from build123d import *

# Parameters (mm, degrees)
SKETCH3_W                                    = 145.5000011
SKETCH3_H                                    = 83.82
BOSS_EXTRUDE1_DEPTH                          = 83.82
SKETCH4_W                                    = 141.50000148
SKETCH4_H                                    = 79.312008
CUT_EXTRUDE1_DEPTH                           = 71.882
CBORE_FOR_M3_HEX_HEAD_CAP_SCREW1_D           = 3.4
CBORE_FOR_M3_HEX_HEAD_CAP_SCREW1_DEPTH       = 3.99999962
CBORE_FOR_M3_HEX_HEAD_CAP_SCREW1_CBORE_D     = 9.351
CBORE_FOR_M3_HEX_HEAD_CAP_SCREW1_CBORE_DEPTH = 2
CUT_EXTRUDE3_REACH                           = 147.5
SKETCH5_R                                    = 12.7
CBORE_FOR_M3_HEX_HEAD_CAP_SCREW2_D           = 3.4
CBORE_FOR_M3_HEX_HEAD_CAP_SCREW2_DEPTH       = 4.507992
CBORE_FOR_M3_HEX_HEAD_CAP_SCREW2_CBORE_D     = 9.351
CBORE_FOR_M3_HEX_HEAD_CAP_SCREW2_CBORE_DEPTH = 2
F_3_0MM_DOWEL_HOLE1_D                        = 3
F_3_0MM_DOWEL_HOLE1_DEPTH                    = 4.507992
F_3_0MM_DOWEL_HOLE2_D                        = 3
F_3_0MM_DOWEL_HOLE2_DEPTH                    = 11.938
CBORE_FOR_M3_HEX_HEAD_CAP_SCREW3_D           = 3.4
CBORE_FOR_M3_HEX_HEAD_CAP_SCREW3_DEPTH       = 11.938
CBORE_FOR_M3_HEX_HEAD_CAP_SCREW3_CBORE_D     = 9.351
CBORE_FOR_M3_HEX_HEAD_CAP_SCREW3_CBORE_DEPTH = 2
SKETCH22_R                                   = 41.75000032
BOSS_EXTRUDE3_DEPTH                          = 170
SKETCH26_R                                   = 36.75001032
CUT_EXTRUDE5_DEPTH                           = 170
SKETCH27_W                                   = 141.50000148
SKETCH27_H                                   = 4.507992
CUT_EXTRUDE7_DEPTH                           = 71.882
SKETCH28_W                                   = 132.727764313
SKETCH28_H                                   = 83.82
CUT_EXTRUDE8_DEPTH                           = 6.35
TAP_DRILL_FOR_M6_TAP2_D                      = 5


with BuildPart() as part:
    # Sketch3 → Boss-Extrude1 (new body)
    with BuildSketch(Plane(origin=(0, 0, 0), x_dir=(1, 0, 0), z_dir=(0, 1, 0))):
        with Locations((33.920258223, -7.464260839)):
            Rectangle(SKETCH3_W, SKETCH3_H)
    extrude(amount=BOSS_EXTRUDE1_DEPTH)

    # Sketch4 → Cut-Extrude1 (cut)
    with BuildSketch(Plane(origin=(0, 83.82, 0), x_dir=(1, 0, 0), z_dir=(0, 1, 0))):
        with Locations((31.920258413, -5.210264839)):
            Rectangle(SKETCH4_W, SKETCH4_H)
    extrude(amount=-CUT_EXTRUDE1_DEPTH, mode=Mode.SUBTRACT)

    # CBORE for M3 Hex Head Cap Screw1
    with Locations(Plane(origin=(106.670258773, 0, 0), x_dir=(0, 0, -1), z_dir=(1, 0, 0))):
        with Locations((-32.411268839, 54.438), (17.588731161, 54.438), (17.588731161, 29.438), (-32.411268839, 29.438)):
            CounterBoreHole(CBORE_FOR_M3_HEX_HEAD_CAP_SCREW1_D / 2, CBORE_FOR_M3_HEX_HEAD_CAP_SCREW1_CBORE_D / 2, CBORE_FOR_M3_HEX_HEAD_CAP_SCREW1_CBORE_DEPTH, depth=CBORE_FOR_M3_HEX_HEAD_CAP_SCREW1_DEPTH)

    # Sketch5 → Cut-Extrude3 (cut, up to next)
    with BuildSketch(Plane(origin=(106.670258773, 0, 0), x_dir=(0, 0, -1), z_dir=(1, 0, 0)), mode=Mode.PRIVATE) as cut_extrude3_sk1:
        with Locations((-7.411268839, 41.938)):
            Circle(SKETCH5_R)
    cut_extrude3_tool1 = extrude(cut_extrude3_sk1.sketch, amount=-CUT_EXTRUDE3_REACH, mode=Mode.PRIVATE) & part.part
    add(cut_extrude3_tool1.solids().sort_by_distance((106.670259, 41.938, 7.411269))[0], mode=Mode.SUBTRACT)

    # CBORE for M3 Hex Head Cap Screw2
    with Locations(Plane.XY.offset(49.374260839)):
        with Locations((100.170259153, 46.938), (100.170259153, 31.938)):
            CounterBoreHole(CBORE_FOR_M3_HEX_HEAD_CAP_SCREW2_D / 2, CBORE_FOR_M3_HEX_HEAD_CAP_SCREW2_CBORE_D / 2, CBORE_FOR_M3_HEX_HEAD_CAP_SCREW2_CBORE_DEPTH, depth=CBORE_FOR_M3_HEX_HEAD_CAP_SCREW2_DEPTH)

    # Ø3.0mm Dowel Hole1
    with Locations(Plane.XY.offset(49.374260839)):
        with Locations((-36.329740847, 46.938), (-36.329740847, 31.938)):
            Hole(F_3_0MM_DOWEL_HOLE1_D / 2, depth=F_3_0MM_DOWEL_HOLE1_DEPTH)

    # Ø3.0mm Dowel Hole2
    with Locations(Plane(origin=(0, 0, 0), x_dir=(-1, 0, 0), z_dir=(0, -1, 0))):
        with Locations((36.329740847, -29.661268839), (36.329740847, -7.411268839), (36.329740847, 14.838731161)):
            Hole(F_3_0MM_DOWEL_HOLE2_D / 2, depth=F_3_0MM_DOWEL_HOLE2_DEPTH)

    # CBORE for M3 Hex Head Cap Screw3
    with Locations(Plane(origin=(0, 0, 0), x_dir=(-1, 0, 0), z_dir=(0, -1, 0))):
        with Locations((-100.170259153, -29.661268839), (-100.170259153, -7.411268839), (-100.170259153, 14.838731161)):
            CounterBoreHole(CBORE_FOR_M3_HEX_HEAD_CAP_SCREW3_D / 2, CBORE_FOR_M3_HEX_HEAD_CAP_SCREW3_CBORE_D / 2, CBORE_FOR_M3_HEX_HEAD_CAP_SCREW3_CBORE_DEPTH, depth=CBORE_FOR_M3_HEX_HEAD_CAP_SCREW3_DEPTH)

    # Sketch22 → Boss-Extrude3 (add)
    with BuildSketch(Plane(origin=(106.670258773, 0, 0), x_dir=(0, 0, -1), z_dir=(1, 0, 0))):
        with Locations((-7.411268839, 41.938)):
            Circle(SKETCH22_R)
    extrude(amount=BOSS_EXTRUDE3_DEPTH)

    # Sketch26 → Cut-Extrude5 (cut)
    with BuildSketch(Plane(origin=(276.670258773, 0, 0), x_dir=(0, 0, -1), z_dir=(1, 0, 0))):
        with Locations((-7.411268839, 41.938)):
            Circle(SKETCH26_R)
    extrude(amount=-CUT_EXTRUDE5_DEPTH, mode=Mode.SUBTRACT)

    # Sketch27 → Cut-Extrude7 (cut)
    with BuildSketch(Plane(origin=(0, 83.82, 0), x_dir=(1, 0, 0), z_dir=(0, 1, 0))):
        with Locations((31.920258413, -47.120264839)):
            Rectangle(SKETCH27_W, SKETCH27_H)
    extrude(amount=-CUT_EXTRUDE7_DEPTH, mode=Mode.SUBTRACT)

    # Sketch28 → Cut-Extrude8 (cut)
    with BuildSketch(Plane(origin=(0, 0, 0), x_dir=(-1, 0, 0), z_dir=(0, -1, 0))):
        with Locations((-27.534139829, -7.464260839)):
            Rectangle(SKETCH28_W, SKETCH28_H)
    extrude(amount=-CUT_EXTRUDE8_DEPTH, mode=Mode.SUBTRACT)

    # Tap Drill for M6 Tap2 (through all)
    with Locations(Plane(origin=(191.670258773, 41.938, -34.338731481), x_dir=(-1, 0, 0), z_dir=(0, 0, -1))):
        with Locations((-28, 0)):
            Hole(TAP_DRILL_FOR_M6_TAP2_D / 2)


solid = part.part
Could you check a few things on this model? Use its own coordinates, in mm. A direction names the side the tool comes from. Coordinates: 2 decimals unless noted, no trailing zeros. Order: outer loops, then holes, each group sorted by start corner. A loop starts at its lowest first (then second) coordinate and runs counter-clockwise, first axis right, second up. Notation, with made-up numbers: (49.25, 28) -> (97.25, 28) arc R18 cw to (97.25, 49) -> close; hole circle Ø3 at (-33.75, -4.5). An arc over 180 degrees is marked (long way). One line per item, written item: value. Start each with the question number.
1) Imagine slicing it at C-C on x = 66.5. List the corners of the cut face in (y, z) for me, plus the area to 3 significant figures.
2) Imagine slicing it at A-A on y = 66.5. List the corners of the cut face in (x, z) for me (3 decimals), plus the area to 3 significant figures.
3) Imagine slicing it at D-D on x = 112. List the corners of the cut face in (y, z) for me.
4) Imagine slicing it at B-B on z = 40.5. List the corners of the cut face in (x, y) for me.
5) If I drill on L1, parallel to Y at x = 10, z = 20.5; L2, parallel to Z at x = 118.5, y = 47; L3, parallel to Z at x = 256, y = 35, over which ranges is the centre line in solid material (lowest first)? Write a range as [from, to].
6) I'm going to push flat-ended pins straight in: pin 1 (4 mm diameter, centred on y = 29.44, z = 32.41, fed in from -X); pin 2 (4 mm diameter, centred on x = -36.33, z = -14.84, fed in from +Y); pin 3 (5.5 mm diameter, centred on x = 100.17, z = 29.66, fed in from -Y). Where does each tip first touch, or does it pass through?
7) Which directions (+Z, -Z, +X, -X, +Y, -Y) give clear straight access to the entire face, cutting with the end or side of a thin tool? Please do faces 1 (the flat face through (28, 6.35, 7)), 2 (the flat face through (98, 2, 7)), 3 (the flat face through (104.67, 27, -18)), 4 (the flat face through (31, 11.938, 7)).
8) We'd pull the mould along Y, two halves only. Please class faces 5 (the flat face through (104.67, 52, 32)), 6 (the flat face through (106, 0, 7)), 7 (the cylindrical face through (190.48, 83.333, 12.846)), 8 (the cylindrical face through (101.184, 0.986, 34.226)): +Y half, -Y half, draft (parallel to the pull), parting line (faces both ways), or undercut.
Answer list:
1. outline: (6.35, -34.45) -> (11.94, -34.45) -> (11.94, 49.37) -> (6.35, 49.37) -> close
1. area: 468 mm2
2. outline: (102.67, -34.446) -> (106.67, -34.446) -> (106.67, -26.349) -> (276.67, -26.349) -> (276.67, -19.925) -> (106.67, -19.925) -> (106.67, 34.748) -> (276.67, 34.748) -> (276.67, 41.172) -> (106.67, 41.172) -> (106.67, 49.374) -> (102.67, 49.374) -> close
2. area: 2,520 mm2
3. outline: circle Ø83.5 at (41.94, 7.41); hole circle Ø73.5 at (41.94, 7.41)
4. outline: (-38.83, 6.35) -> (93.9, 6.35) -> (93.9, 0) -> (106.67, 0) -> (106.67, 16.48) -> (276.67, 16.48) -> (276.67, 25.95) -> (106.67, 25.95) -> (106.67, 57.93) -> (276.67, 57.93) -> (276.67, 67.4) -> (106.67, 67.4) -> (106.67, 83.82) -> (102.67, 83.82) -> (102.67, 11.94) -> (-38.83, 11.94) -> close
5. L1: y = [6.35, 11.94]
5. L2: z = [-34.03, -28.99], [43.81, 48.85]
5. L3: z = [-33.76, -28.68], [43.5, 48.58]
6. pin 1: stops at x = 102.67
6. pin 2: stops at y = 11.94
6. pin 3: stops at y = 2
7. face 1: +Z, -Z, -X, -Y
7. face 2: -Y
7. face 3: +X
7. face 4: +Z, -Z, -X, +Y
8. face 5: undercut
8. face 6: -Y half
8. face 7: parting line
8. face 8: draft
